```python
from build123d import *

# Parameters (mm, degrees)
SKETCH1_R           = 1.55
BOSS_EXTRUDE1_DEPTH = 10
SKETCH2_W           = 10.5
SKETCH2_H           = 145
CUT_EXTRUDE1_DEPTH  = 5
SKETCH3_W           = 12
SKETCH3_H           = 25
CUT_EXTRUDE2_DEPTH  = 181.969610709
SKETCH4_W           = 50
SKETCH4_H           = 3
CUT_EXTRUDE3_DEPTH  = 5
FILLET1_R           = 3
SKETCH6_R           = 1.55
CUT_EXTRUDE4_DEPTH  = 5
CHAMFER2_SIZE       = 1
SKETCH7_W           = 3
SKETCH7_H           = 3
CUT_EXTRUDE5_DEPTH  = 12
SKETCH8_W           = 3
SKETCH8_H           = 3
CUT_EXTRUDE6_DEPTH  = 181.828648173


with BuildPart() as part:
    # Sketch1 → Boss-Extrude1 (new body)
    with BuildSketch(Plane(origin=(0, 0, 0), x_dir=(1, 0, 0), z_dir=(0, 1, 0))):
        with BuildLine():
            Line((0, -30), (0, 0))
            Line((0, 0), (-45, 0))
            Line((-45, 0), (-45, -10))
            Line((-45, -10), (-20, -55))
            Line((-20, -55), (-20, -175))
            Line((-20, -175), (0, -175))
            Line((0, -175), (0, -165))
            ThreePointArc((0, -165), (-2.828427125, -163.828427125), (-4, -161))
            Line((-4, -161), (-4, -34))
            ThreePointArc((-4, -34), (-2.828427125, -31.171572875), (0, -30))
        make_face()
        with Locations(Location((-40, -5, 0), (0, 0, 270))):
            Circle(SKETCH1_R, mode=Mode.SUBTRACT)
    boss_extrude1 = extrude(amount=BOSS_EXTRUDE1_DEPTH)

    # Sketch2 → Cut-Extrude1 (cut)
    with BuildSketch(Plane(origin=(0, 10, 0), x_dir=(1, 0, 0), z_dir=(0, 1, 0))):
        with Locations((-5.25, -97.5)):
            Rectangle(SKETCH2_W, SKETCH2_H)
    cut_extrude1 = extrude(amount=-CUT_EXTRUDE1_DEPTH, mode=Mode.SUBTRACT)

    # Mirror1: Boss-Extrude1, Cut-Extrude1 across plane
    add(boss_extrude1.mirror(Plane(origin=(0, 0, 0), x_dir=(0, 0, 1), z_dir=(1, 0, 0))))
    add(cut_extrude1.mirror(Plane(origin=(0, 0, 0), x_dir=(0, 0, 1), z_dir=(1, 0, 0))), mode=Mode.SUBTRACT)

    # Sketch3 → Cut-Extrude2 (cut, through all)
    with BuildSketch(Plane(origin=(0, 10, 0), x_dir=(1, 0, 0), z_dir=(0, 1, 0))):
        with Locations((0, -12.5)):
            Rectangle(SKETCH3_W, SKETCH3_H)
    extrude(amount=-CUT_EXTRUDE2_DEPTH, mode=Mode.SUBTRACT)

    # Sketch4 → Cut-Extrude3 (cut)
    with BuildSketch(Plane(origin=(0, 10, 0), x_dir=(1, 0, 0), z_dir=(0, 1, 0))):
        with Locations((0, -10)):
            Rectangle(SKETCH4_W, SKETCH4_H)
    extrude(amount=-CUT_EXTRUDE3_DEPTH, mode=Mode.SUBTRACT)

    # Fillet1
    fillet1_edges = [part.edges().sort_by_distance(p)[0] for p in [
        (-25.5, 10, 0),
        (25.5, 10, 0),
        (-32.5, 10, 32.5),
        (-20, 10, 115),
        (0, 10, 175),
        (20, 10, 115),
        (32.5, 10, 32.5),
    ]]
    fillet(fillet1_edges, radius=FILLET1_R)

    # Sketch6 → Cut-Extrude4 (cut)
    # profile 1 of 2: a face of its own
    with BuildSketch(Plane.XZ):
        Polygon((-42.416024464, 2.82621855), (-39.325462274, 1.820770713), (-36.90943781, 3.994552163), (-37.583975536, 7.17378145), (-40.674537726, 8.179229287), (-43.09056219, 6.005447837), align=None)
        with Locations(Location((-40, 5, 0), (0, 0, 270))):
            Circle(SKETCH6_R, mode=Mode.SUBTRACT)
    # profile 2 of 2: a face of its own
    with BuildSketch(Plane.XZ):
        Polygon((36.81146344, 4.370925598), (38.950526133, 1.924109137), (42.139062693, 2.553183539), (43.18853656, 5.629074402), (41.049473867, 8.075890863), (37.860937307, 7.446816461), align=None)
        with Locations(Location((40, 5, 0), (0, 0, 270))):
            Circle(SKETCH6_R, mode=Mode.SUBTRACT)
    extrude(amount=-CUT_EXTRUDE4_DEPTH, mode=Mode.SUBTRACT)

    # Chamfer2
    chamfer2_edges = [part.edges().sort_by_distance(p)[0] for p in [
        (-40.870743369, 5, 2.323494632),
        (-42.753293327, 5, 4.415833194),
        (-41.882549958, 5, 7.092338562),
        (-39.129256631, 5, 7.676505368),
        (-37.246706673, 5, 5.584166806),
        (-38.117450042, 5, 2.907661438),
        (37.880994786, 5, 3.147517367),
        (37.336200373, 5, 5.908871029),
        (39.455205587, 5, 7.761353662),
        (42.119005214, 5, 6.852482633),
        (42.663799627, 5, 4.091128971),
        (40.544794413, 5, 2.238646338),
    ]]
    chamfer(chamfer2_edges, length=CHAMFER2_SIZE)

    # Sketch7 → Cut-Extrude5 (cut)
    with BuildSketch(Plane.XY.offset(175)):
        with Locations((0, 8.5)):
            Rectangle(SKETCH7_W, SKETCH7_H)
        with Locations((0, 1.5)):
            Rectangle(SKETCH7_W, SKETCH7_H)
    extrude(amount=-CUT_EXTRUDE5_DEPTH, mode=Mode.SUBTRACT)

    # Sketch8 → Cut-Extrude6 (cut, through all)
    with BuildSketch(Plane(origin=(0, 7, 0), x_dir=(1, 0, 0), z_dir=(0, 1, 0))):
        with Locations((0, -173.5)):
            Rectangle(SKETCH8_W, SKETCH8_H)
    extrude(amount=-CUT_EXTRUDE6_DEPTH, mode=Mode.SUBTRACT)


solid = part.part
```
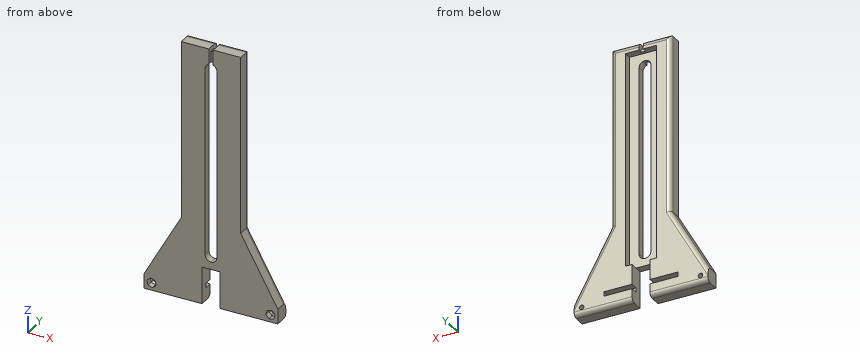
The listing builds one solid part. Answer for the finished solid, in the listing's coordinates (mm). Round coordinates to 2 decimals unless told otherwise and drop trailing zeros. Loops run counter-clockwise (first coordinate to the right, second up) from the corner with the lowest first, then second, coordinate; pieces in that order, holes last.
1) A cutting plane is placed at A-A on z = 136. Determine the outline of the cut face in (x, y).
Outcome:
outline: (-20, 0) - (-4, 0) - (-4, 5) - (-10.5, 5) - (-10.5, 10) - (-17, 10) arc R3 ccw to (-20, 7) - close; (4, 0) - (20, 0) - (20, 7) arc R3 ccw to (17, 10) - (10.5, 10) - (10.5, 5) - (4, 5) - close
2) Consider line 1 (X direction, y = 8.8, z = 5); line 2 (X direction, y = 2, z = 134.5); line 3 (Z direction, x = -9.5, y = 9.5). Determine where each line is inside the solid, lowest interval first.
Outcome:
line 1: x = -45 to -41.55, -38.45 to -6, 6 to 38.45, 41.55 to 45
line 2: x = -20 to -4, 4 to 20
line 3: z = 1.34 to 8.5, 11.5 to 25, 170 to 173.66
3) A cutting plane is placed at B-B on y = 1.5. Give the number of separate pieces and of enclosed holes in the cut face, plus the area to 3 significant figures.
Outcome:
separate pieces: 1
enclosed holes: 2
area: 7,170 mm2
4) Given P1, Ø2.5, axis at y = 7.5, z = 63.5, coming from the -X side; P2, Ø4, axis at y = 3, z = 85, coming from the +X side; P3, Ø1.5, axis at x = 19, y = 8.5, coming from the -Z side, each flat-ended and moving along its own axis, determine where each tip first touches the part or whether it passes through.
Outcome:
P1: stops at x = -20
P2: stops at x = 20
P3: stops at z = 0.1
